Here's how the part is built. I have some questions about the finished solid (model axes, mm). A direction names the side the tool comes from. Round coordinates to 2 decimals unless told otherwise and drop trailing zeros. Write each loop counter-clockwise with the first axis right and the second up, starting at its lowest first coordinate (ties: lowest second). Pieces come first, ordered by that corner, then holes. Notation, with made-up numbers: (25, 62.5) - (52, 62.5) arc R18 cw to (52, 66.5) - close; hole circle Ø11 at (46, 87.5). An arc over 180 degrees is marked (long way). One line per question, with ' | ' between items. Start each with the question number.
(1) Will these pins go through, and if not, where does the flat tip stop? pin 1 (0.9 mm diameter, centred on y = 6, z = 3, fed in from +X); pin 2 (1.2 mm diameter, centred on x = -30.75, y = -10.03, fed in from -Z); pin 3 (3.5 mm diameter, centred on x = 6.5, y = -7.5, fed in from +Z); pin 4 (1.5 mm diameter, centred on y = 1.5, z = -5.5, fed in from +X).
(2) Imagine slicing it at C-C (x = -30.75). Write out the boundary of the cut face in (y, z) (3 decimals).
(3) If I drill on L1, parallel to X at y = 3, z = -9; L2, parallel to Y at x = 5.5, z = -11.7; L3, parallel to X at y = 0.75, z = -3, over which ranges is the centre line in solid material (lowest first)?
(4) Thinking about a two-plate mould opening in Y: for faces 1 (the flat face through (-5, 3.25, -6)), 2 (the flat face through (-5, -9, -10.5)), 3 (the flat face through (30, 11, 6)), which applies, pulls with the +Y half, pulls with the -Y half, needs draft (parallel to the pull), parting line crosses it, or undercut?
(5) Imagine slicing it at D-D (x = 5.5). Write out the boundary of the cut face in (y, z), plus the area to 3 significant figures.
(6) For faces 4 (the flat face through (-2.35, -6, -6)), 5 (the flat face through (-3, -14.75, -2)), 6 (the flat face through (30.72, 7.1, 4.47)), 7 (the cylindrical face through (5.2, -5.47, -4.16)), which set-ups out of +Z, -Z, +X, -X, +Y, -Y let a thin tool reach every point of the face, with its end or its side?
(7) Imagine slicing it at B-B (y = 10.03). Write out the boundary of the cut face in (x, z) (3 decimals), plus the area to 3 significant figures.
(8) Imagine slicing it at A-A (z = -3.25). Write out the boundary of the cut face in (x, y), plus the area to 3 significant figures.
from build123d import *

# Parameters (mm, degrees)
BOSS_EXTRUDE1_DEPTH = 2
SKETCH5_R           = 2.6
BOSS_EXTRUDE4_DEPTH = 4
SKETCH6_R           = 1.025
CUT_EXTRUDE1_DEPTH  = 39.907743445
BOSS_EXTRUDE6_DEPTH = 4
CHAMFER1_SIZE       = 5
SKETCH8_W           = 6.3
SKETCH8_H           = 18
BOSS_EXTRUDE8_DEPTH = 12
SKETCH9_R           = 1.05
CUT_EXTRUDE3_DEPTH  = 41.912253666
SKETCH10_R          = 2.3
CUT_EXTRUDE4_DEPTH  = 12.5


with BuildPart() as part:
    # Sketch1 → Boss-Extrude1 (new body)
    with BuildSketch(Plane.XY):
        Polygon((-33.5, 14.75), (-35.5, 12.75), (-35.5, -12.75), (-33.5, -14.75), (33.5, -14.75), (35.5, -12.75), (35.5, 12.75), (33.5, 14.75), align=None)
    extrude(amount=BOSS_EXTRUDE1_DEPTH)

    # Sketch5 → Boss-Extrude4 (add)
    with BuildSketch(Plane.XY.offset(2)):
        with Locations(Location((-30.75, 10.03, 0), (0, 0, 180))):
            Circle(SKETCH5_R)
        with Locations(Location((30.75, 10.03, 0), (0, 0, 180))):
            Circle(SKETCH5_R)
        with Locations(Location((30.75, -10.03, 0), (0, 0, 180))):
            Circle(SKETCH5_R)
        with Locations(Location((-30.75, -10.03, 0), (0, 0, 180))):
            Circle(SKETCH5_R)
    extrude(amount=BOSS_EXTRUDE4_DEPTH)

    # Sketch6 → Cut-Extrude1 (cut, through all)
    with BuildSketch(Plane.XY.offset(6)):
        with Locations((-30.75, 10.03)):
            Circle(SKETCH6_R)
        with Locations(Location((30.75, 10.03, 0), (0, 0, 180))):
            Circle(SKETCH6_R)
        with Locations((30.75, -10.03)):
            Circle(SKETCH6_R)
        with Locations(Location((-30.75, -10.03, 0), (0, 0, 180))):
            Circle(SKETCH6_R)
    extrude(amount=-CUT_EXTRUDE1_DEPTH, mode=Mode.SUBTRACT)

    # Sketch7 → Boss-Extrude6 (add)
    with BuildSketch(Plane.XY.offset(2)):
        with BuildLine():
            Line((-31.75, 7.63), (-31.75, 3.63))
            Line((-31.75, 3.63), (-29.75, 3.63))
            Line((-29.75, 3.63), (-29.75, 7.63))
            ThreePointArc((-29.75, 7.63), (-30.75, 7.43), (-31.75, 7.63))
        make_face()
        with BuildLine():
            Line((29.75, 7.63), (29.75, 3.63))
            Line((29.75, 3.63), (31.75, 3.63))
            Line((31.75, 3.63), (31.75, 7.63))
            ThreePointArc((31.75, 7.63), (30.75, 7.43), (29.75, 7.63))
        make_face()
    extrude(amount=BOSS_EXTRUDE6_DEPTH)

    # Chamfer1
    # the kernel refuses this chamfer: 5 mm, written as the material it takes off along each edge
    with BuildSketch(Plane(origin=(16.89158506, 3.63, 6), x_dir=(0, 0.9996219169112968, 0.027495876610586317), z_dir=(1, 0, 0))) as chamfer1_piece_1_section:
        Polygon((CHAMFER1_SIZE * 0.999621916911, -CHAMFER1_SIZE * 0.0274958766106), (-CHAMFER1_SIZE * 0.0274958766106, -CHAMFER1_SIZE * 0.999621916911), (0, 0), align=None)
    chamfer1_piece_1 = extrude(amount=27.71682988, mode=Mode.PRIVATE)
    chamfer1_piece_1 = split(chamfer1_piece_1, bisect_by=Plane(origin=(30.75, 5.358592062, 2), z_dir=(0, 0, 1)), keep=Keep.TOP, mode=Mode.PRIVATE)
    add(chamfer1_piece_1, mode=Mode.SUBTRACT)
    with BuildSketch(Plane(origin=(-44.60841494, 3.63, 6), x_dir=(0, 0.9996219169112968, 0.027495876610586317), z_dir=(1, 0, 0))) as chamfer1_piece_2_section:
        Polygon((CHAMFER1_SIZE * 0.999621916911, -CHAMFER1_SIZE * 0.0274958766106), (-CHAMFER1_SIZE * 0.0274958766106, -CHAMFER1_SIZE * 0.999621916911), (0, 0), align=None)
    chamfer1_piece_2 = extrude(amount=27.71682988, mode=Mode.PRIVATE)
    chamfer1_piece_2 = split(chamfer1_piece_2, bisect_by=Plane(origin=(-30.75, 5.358592062, 2), z_dir=(0, 0, 1)), keep=Keep.TOP, mode=Mode.PRIVATE)
    add(chamfer1_piece_2, mode=Mode.SUBTRACT)

    # Sketch8 → Boss-Extrude8 (add)
    with BuildSketch(Plane(origin=(0, 0, 0), x_dir=(-1, 0, 0), z_dir=(0, 0, -1))):
        with Locations((-5.5, -5.75)):
            Rectangle(SKETCH8_W, SKETCH8_H)
        with Locations((5.5, -5.75)):
            Rectangle(SKETCH8_W, SKETCH8_H)
    extrude(amount=BOSS_EXTRUDE8_DEPTH)

    # Sketch9 → Cut-Extrude3 (cut, through all)
    with BuildSketch(Plane.XY.offset(2)):
        with Locations((5.5, -7.75)):
            Circle(SKETCH9_R)
        with Locations((5.5, -0.75)):
            Circle(SKETCH9_R)
        with Locations(Location((-5.5, -0.75, 0), (0, 0, 180))):
            Circle(SKETCH9_R)
        with Locations(Location((-5.5, -7.75, 0), (0, 0, 180))):
            Circle(SKETCH9_R)
    extrude(amount=-CUT_EXTRUDE3_DEPTH, mode=Mode.SUBTRACT)

    # Sketch10 → Cut-Extrude4 (cut)
    with BuildSketch(Plane.XY.offset(2)):
        with Locations((5.5, -7.75)):
            Circle(SKETCH10_R)
        with Locations((5.5, -0.75)):
            Circle(SKETCH10_R)
        with Locations(Location((-5.5, -0.75, 0), (0, 0, 180))):
            Circle(SKETCH10_R)
        with Locations(Location((-5.5, -7.75, 0), (0, 0, 180))):
            Circle(SKETCH10_R)
    extrude(amount=-CUT_EXTRUDE4_DEPTH, mode=Mode.SUBTRACT)


solid = part.part
Check sheet entries:
1) pin 1: x = 31.75 | pin 2: through | pin 3: z = 2 | pin 4: x = 8.65
2) outline: (-14.75, 0) - (-11.055, 0) - (-11.055, 6) - (-12.63, 6) - (-12.63, 2) - (-14.75, 2) - close; (-9.005, 0) - (9.005, 0) - (9.005, 6) - (8.63, 6) - (4.63, 2) - (-7.43, 2) - (-7.43, 6) - (-9.005, 6) - close; (11.055, 0) - (14.75, 0) - (14.75, 2) - (12.63, 2) - (12.63, 6) - (11.055, 6) - close
3) L1: -8.65 to -2.35, 2.35 to 8.65 | L2: -14.75 to -8.8, -6.7 to -1.8, 0.3 to 3.25 | L3: -8.65 to -7.24, -3.76 to -2.35, 2.35 to 3.76, 7.24 to 8.65
4) face 1: pulls with the +Y half | face 2: undercut | face 3: needs draft
5) outline: (-14.75, -12) - (-8.8, -12) - (-8.8, -10.5) - (-10.05, -10.5) - (-10.05, 2) - (-14.75, 2) - close; (-6.7, -12) - (-1.8, -12) - (-1.8, -10.5) - (-3.05, -10.5) - (-3.05, 2) - (-5.45, 2) - (-5.45, -10.5) - (-6.7, -10.5) - close; (0.3, -12) - (3.25, -12) - (3.25, 0) - (14.75, 0) - (14.75, 2) - (1.55, 2) - (1.55, -10.5) - (0.3, -10.5) - close | area: 154 mm^2
6) face 4: -Z, +Y, -Y | face 5: +Z, -Z, +X, -X, -Y | face 6: +Z, +X, -X | face 7: +Z
7) outline: (-35.5, 0) - (-31.775, 0) - (-31.775, 6) - (-33.35, 6) - (-33.35, 2) - (-35.5, 2) - close; (-29.725, 0) - (29.725, 0) - (29.725, 6) - (28.15, 6) - (28.15, 2) - (-28.15, 2) - (-28.15, 6) - (-29.725, 6) - close; (31.775, 0) - (35.5, 0) - (35.5, 2) - (33.35, 2) - (33.35, 6) - (31.775, 6) - close | area: 159 mm^2
8) outline: (-8.65, -14.75) - (-2.35, -14.75) - (-2.35, 3.25) - (-8.65, 3.25) - close; (2.35, -14.75) - (8.65, -14.75) - (8.65, 3.25) - (2.35, 3.25) - close; hole circle Ø4.6 at (-5.5, -7.75); hole circle Ø4.6 at (-5.5, -0.75); hole circle Ø4.6 at (5.5, -7.75); hole circle Ø4.6 at (5.5, -0.75) | area: 160 mm^2
